CAD build for the part. Positions are in the model's coordinates, mm. A direction names the side the tool comes from. Coordinates: 2 decimals unless noted, no trailing zeros. Order: outer loops, then holes, each group sorted by start corner. A loop starts at its lowest first (then second) coordinate and runs counter-clockwise, first axis right, second up.
from build123d import *
from build123d.topology import SkipClean

# Parameters (mm, degrees)
BOSS_EXTRUDE1_DEPTH = 96.52
SKETCH2_R           = 9.525
BOSS_EXTRUDE2_DEPTH = 3.81
CUT_EXTRUDE1_DEPTH  = 1.27
CUT_EXTRUDE2_START  = -114.3
CUT_EXTRUDE2_DEPTH  = 16.51


with BuildPart() as part:
    # Sketch1 → Boss-Extrude1 (new, symmetric)
    with BuildSketch(Plane(origin=(0, 0, 0), x_dir=(1, 0, 0), z_dir=(0, 1, 0))):
        with BuildLine():
            ThreePointArc((-9.525, -60.325), (-6.735192091, -67.060192091), (0, -69.85))
            ThreePointArc((0, -69.85), (6.735192091, -67.060192091), (9.525, -60.325))
            Line((9.525, -60.325), (9.525, 69.85))
            Line((9.525, 69.85), (-9.525, 69.85))
            Line((-9.525, 69.85), (-9.525, -60.325))
        make_face()
    extrude(amount=BOSS_EXTRUDE1_DEPTH, both=True)

    # Sketch2 → Boss-Extrude2 (add)
    with SkipClean():  # the faces are left unmerged after this step: merging them gives an invalid solid
        with BuildSketch(Plane.XZ.offset(96.52)):
            with Locations(Location((0, 60.325, 0), (0, 0, 270))):
                Circle(SKETCH2_R)
        extrude(amount=BOSS_EXTRUDE2_DEPTH)

    # Sketch3 → Cut-Extrude1 (cut)
    with SkipClean():  # the faces are left unmerged after this step: merging them gives an invalid solid
        with BuildSketch(Plane(origin=(0, 96.52, 0), x_dir=(1, 0, 0), z_dir=(0, 1, 0))):
            with BuildLine():
                Line((-2.653910055, -58.137819903), (-2.000444386, -46.187796735))
                ThreePointArc((-2.000444386, -46.187796735), (-0.003346519, -44.297000013), (1.993597371, -46.187959354))
                Line((1.993597371, -46.187959354), (2.646089941, -58.138035694))
                ThreePointArc((2.646089941, -58.138035694), (-0.004140468, -63.796999997), (-2.653910055, -58.137819903))
            make_face()
        extrude(amount=-CUT_EXTRUDE1_DEPTH, mode=Mode.SUBTRACT)

    # Sketch5 → Cut-Extrude2 (cut)
    with SkipClean():  # the faces are left unmerged after this step: merging them gives an invalid solid
        with BuildSketch(Plane.XZ.offset(96.52).offset(CUT_EXTRUDE2_START)):
            with BuildLine():
                Line((9.525, 44.45), (-9.525, 44.45))
                Line((-9.525, 44.45), (-9.525, 60.325))
                ThreePointArc((-9.525, 60.325), (0, 50.8), (9.525, 60.325))
                Line((9.525, 60.325), (9.525, 44.45))
            make_face()
        extrude(amount=CUT_EXTRUDE2_DEPTH, mode=Mode.SUBTRACT)


solid = part.part
1) Pin check, flat tips, straight feed: P1, Ø5.5, axis at x = 4, z = 17, coming from the -Y side; P2, Ø5.5, axis at x = -1, z = 57, coming from the +Y side. Stop position of each tip, or through.
2) Two-plate mould, pull along X, no slides. Class faces 3 (the flat face through (0, 95.25, 54)), 4 (the flat face through (-9.525, 1, -6)), 5 (the flat face through (0, 10, 44.45)): released by +X, released by -X, zero draft, split by the parting line, or undercut.
3) Slice it at B-B (y = 10). List the corners of the cut face in (x, z) (3 decimals).
4) Drill centre lines: probe 1 along Y at (x, z) = (-6.25, 45.5); probe 2 along Y at (x, z) = (2.75, 10); probe 3 along Z at (x, y) = (2, 76). Where is each one in solid material? Low to high.
5) Which spindle directions (+Z, -Z, +X, -X, +Y, -Y) get a long thin tool onto all of the face, cutting with end or side? Do faces 1 (the flat face through (0, 96.52, -1)), 2 (the cylindrical face through (0.105, 95.894, 63.795)). Say none if no direction does.
6) Slice it at C-C (z = -17). List the corners of the cut face in (x, y) (3 decimals).
7) Slice it at A-A (x = 0). List the corners of the cut face in (y, z).
Worked out:
1. P1: stops at y = -96.52
1. P2: stops at y = 96.52
2. face 3: undercut
2. face 4: released by -X
2. face 5: zero draft
3. outline: (-9.525, -69.85) - (9.525, -69.85) - (9.525, 44.45) - (-9.525, 44.45) - close; circle Ø19.05 at (0, 60.325)
4. probe 1: y = -96.52 to 1.27, 17.78 to 96.52
4. probe 2: y = -96.52 to 96.52
4. probe 3: z = -69.85 to 69.64
5. face 1: +Z, -Z, +X, -X, +Y
5. face 2: +Y
6. outline: (-9.525, -96.52) - (9.525, -96.52) - (9.525, 96.52) - (-9.525, 96.52) - close
7. outline: (-100.33, 50.8) - (-96.52, 50.8) - (-96.52, -69.85) - (96.52, -69.85) - (96.52, 44.3) - (95.25, 44.3) - (95.25, 63.8) - (96.52, 63.8) - (96.52, 69.85) - (-100.33, 69.85) - close; hole (1.27, 44.45) - (17.78, 44.45) - (17.78, 50.8) - (1.27, 50.8) - close
